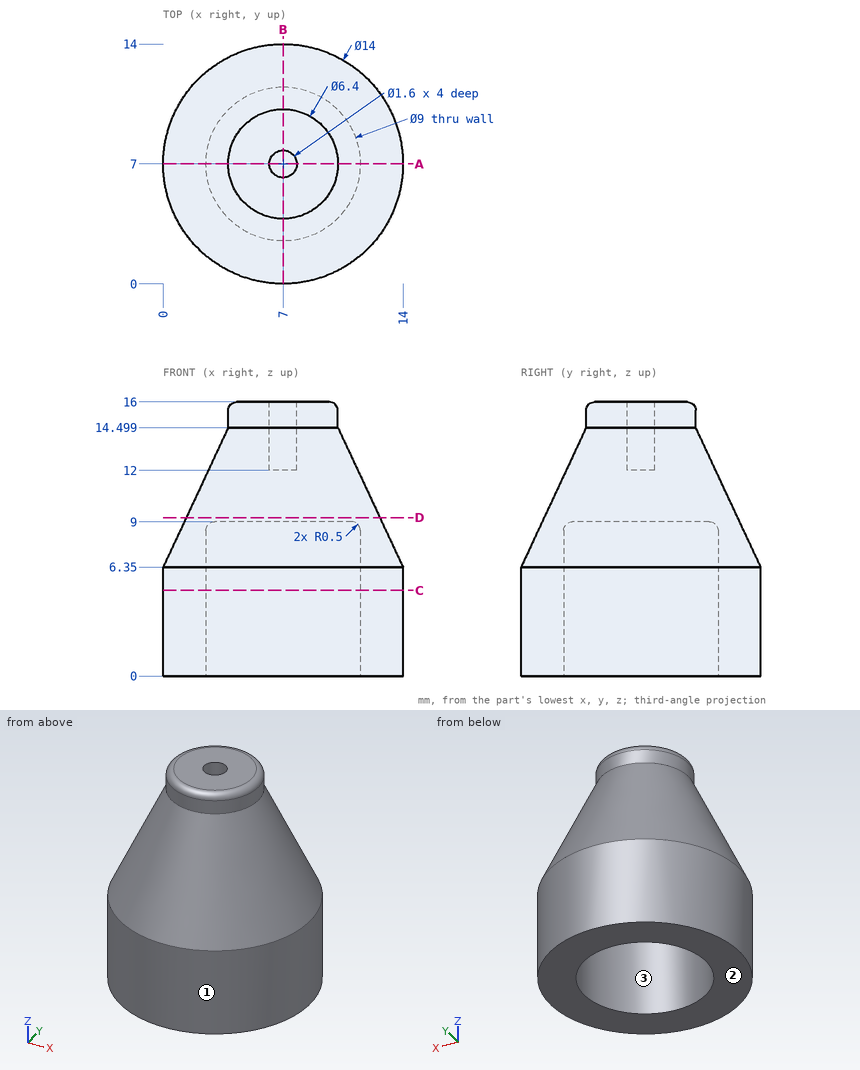
Part print with two shaded views. Sizes in mm from the minimum x, y, z corner. Give positions to 0.01 mm unless a question says otherwise; leave off trailing zeros. Order: outer loops, then holes, each group sorted by start corner. A loop starts at its lowest first (then second) coordinate and runs counter-clockwise, first axis right, second up. Notation, with made-up numbers: M 13.5,73 L 22.5,73 A9 cw 22.5,88 Z; hole C 47.5,-5 d10. An arc over 180 degrees is marked long. Write item = value, one per line.
Q1. Drill centre lines: line 1 (X direction, y = 7, z = 15); line 2 (X direction, y = 7, z = 2); line 3 (Y direction, x = 6.5, z = 2). Where is each one in solid material? Low to high. Write a range as [from, to].
Derived:
line_1 = [3.8, 6.2], [7.8, 10.2]
line_2 = [0, 2.5], [11.5, 14]
line_3 = [0.02, 2.53], [11.47, 13.98]
Q2. Cut at D-D, the plane z = 9.25. List the corners of the cut face in (x, y) (1 decimal), then the cut area to 3 significant figures.
Derived:
outline = C 7,7 d11.3
area = 100 mm2
Q3. Flat gauge pins, fed straight in: pin 1 (0.5 mm diameter, centred on x = 6.5, y = 7, fed in from +Z); pin 2 (1 mm diameter, centred on y = 4, z = 4, fed in from +X); pin 3 (2 mm diameter, centred on y = 7, z = 14, fed in from -X). Where does each tip first touch, or does it go through?
Derived:
pin_1 = 12
pin_2 = 13.54
pin_3 = 3.1
Q4. Cut at C-C, the plane z = 5. List the corners of the cut face in (x, y).
Derived:
outline = C 7,7 d14; hole C 7,7 d9
Q5. Two-plate mould, pull along X, no slides. Class the marked faces 1, 2 and 3: pulls with the +X half, pulls with the -X half, needs draft (parallel to the pull), parting line crosses it, or undercut.
Derived:
face_1 = parting line crosses it
face_2 = needs draft
face_3 = undercut
Q6. Cut at A-A, the plane y = 7. List the corners of the cut face in (x, z).
Derived:
outline = M 0,0 L 2.5,0 L 2.5,8.5 A0.5 cw 3,9 L 11,9 A0.5 cw 11.5,8.5 L 11.5,0 L 14,0 L 14,6.35 L 10.2,14.5 L 10.2,15.5 A0.5 ccw 9.7,16 L 7.8,16 L 7.8,12 L 6.2,12 L 6.2,16 L 4.3,16 A0.5 ccw 3.8,15.5 L 3.8,14.5 L 0,6.35 Z
